Source: CAD feature listing. Evaluate the final solid. Frame: model axes, mm. Face numbers are marked on the shaded views. Give positions to 0.01 mm unless a question says otherwise; leave off trailing zeros. Write item = value, one per line.
from build123d import *

# Parameters (mm, degrees)
F1_DEPTH = 10
F2_DEPTH = 2.5
F3_R     = 5
F5_DEPTH = 12.501
F6_SIZE  = 1.5


# Not quite as in the source:
# - ends of sketch curves that miss each other by under 0.0002 mm in the source are joined


with BuildPart() as f1:
    # F0 (on Top) → F1 (new body, symmetric)
    with BuildSketch(Plane.XY):
        with BuildLine():
            ThreePointArc((-61.1270550584, 5.6233035221), (-64.3120758187, 10.4909176924), (-69.1094465162, 13.7807899309))
            ThreePointArc((-69.1094465162, 13.7807899309), (-89.3390658482, 4.5099582499), (-78.083775001, -14.6865061725))
            ThreePointArc((-78.083775001, -14.6865061725), (-72.0748340452, -14.7053930071), (-66.5406341793, -12.3643761411))
            ThreePointArc((-66.5406341793, -12.3643761411), (-71.7812655501, -10.9856736162), (-77.0668876123, -9.7910032715))
            ThreePointArc((-77.0668876123, -9.7910032715), (-84.570415019, 3.0066388333), (-71.0840021309, 9.1871932872))
            ThreePointArc((-71.0840021309, 9.1871932872), (-66.1610088951, 7.2502451775), (-61.1270550584, 5.6233035221))
        make_face()
        with BuildLine():
            ThreePointArc((-60.0331133604, 0), (-60.3091384465, 2.8643607899), (-61.1270550584, 5.6233035221))
            ThreePointArc((-61.1270550584, 5.6233035221), (-66.1610088951, 7.2502451775), (-71.0840021309, 9.1871932872))
            ThreePointArc((-71.0840021309, 9.1871932872), (-66.6817328669, 5.5004039718), (-65.0331133604, 0))
            ThreePointArc((-65.0331133604, 0), (-68.7219226752, -7.7568596826), (-77.0668877875, -9.791004115))
            ThreePointArc((-77.0668877875, -9.791004115), (-71.7812655501, -10.9856736162), (-66.5406341793, -12.3643761411))
            ThreePointArc((-66.5406341793, -12.3643761411), (-61.7593198612, -6.9861581818), (-60.0331133604, 0))
        make_face()
        with BuildLine():
            ThreePointArc((-13.906058302, 5.6233035221), (-8.2506059576, -12.5270707403), (10.6578947368, -10.5550594398))
            ThreePointArc((10.6578947368, -10.5550594398), (10.1646331199, -5.2877713941), (10, 0))
            ThreePointArc((10, 0), (-5.5004039718, -8.3513804935), (-3.9491112295, 9.1871932872))
            ThreePointArc((-3.9491112295, 9.1871932872), (-8.8721044653, 7.2502451775), (-13.906058302, 5.6233035221))
        make_face()
        with BuildLine():
            ThreePointArc((10.6578947368, -10.5550594398), (13.8720658348, -5.7066443269), (15, 0))
            ThreePointArc((15, 0), (8.2506059576, 12.5270707403), (-5.9236668442, 13.7807899309))
            ThreePointArc((-5.9236668442, 13.7807899309), (-10.7210375417, 10.4909176924), (-13.906058302, 5.6233035221))
            ThreePointArc((-13.906058302, 5.6233035221), (-8.8721044653, 7.2502451775), (-3.9491112295, 9.1871932872))
            ThreePointArc((-3.9491112295, 9.1871932872), (5.5004039718, 8.3513804935), (10, 0))
            ThreePointArc((10, 0), (10.1646331199, -5.2877713941), (10.6578947368, -10.5550594398))
        make_face()
        with BuildLine():
            ThreePointArc((26.5285242746, -50.3652361455), (23.527969189, -46.0081385383), (20.8042767721, -41.4728182632))
            ThreePointArc((20.8042767721, -41.4728182632), (9.3957138654, -44.3489563966), (3.5718338704, -54.5719647583))
            ThreePointArc((3.5718338704, -54.5719647583), (7.2428277606, -58.5580457504), (10.7722421784, -62.6700126379))
            ThreePointArc((10.7722421784, -62.6700126379), (12.3181130698, -48.4091450465), (26.5285242746, -50.3652361455))
        make_face()
        with BuildLine():
            ThreePointArc((33.4730565422, -56.2905580449), (32.7252146942, -51.6133806899), (30.5562581408, -47.4025751957))
            ThreePointArc((30.5562581408, -47.4025751957), (26.2662839534, -43.4739435732), (20.8042767721, -41.4728182632))
            ThreePointArc((20.8042767721, -41.4728182632), (23.527969189, -46.0081385383), (26.5285242746, -50.3652361455))
            ThreePointArc((26.5285242746, -50.3652361455), (27.9744953102, -53.1724398082), (28.4730565422, -56.2905580449))
            ThreePointArc((28.4730565422, -56.2905580449), (21.8636206345, -65.6982184946), (10.772241515, -62.6700131875))
            ThreePointArc((10.772241515, -62.6700131875), (7.2428277606, -58.5580457504), (3.5718338704, -54.5719647583))
            ThreePointArc((3.5718338704, -54.5719647583), (4.0929857429, -60.5582932532), (6.9218340013, -65.8597407588))
            ThreePointArc((6.9218340013, -65.8597407588), (23.5589026806, -70.4020487194), (33.4730565422, -56.2905580449))
        make_face()
        with BuildLine():
            ThreePointArc((-66.5406341793, -12.3643761411), (-72.0748340452, -14.7053930071), (-78.083775001, -14.6865061725))
            ThreePointArc((-78.083775001, -14.6865061725), (-31.2272831079, -33.0410645358), (6.9218340013, -65.8597407588))
            ThreePointArc((6.9218340013, -65.8597407588), (4.0929857429, -60.5582932532), (3.5718338704, -54.5719647583))
            ThreePointArc((3.5718338704, -54.5719647583), (-28.6485123869, -28.7573803523), (-66.5406341793, -12.3643761411))
        make_face()
        with BuildLine():
            ThreePointArc((-13.906058302, 5.6233035221), (-10.7210375417, 10.4909176924), (-5.9236668442, 13.7807899309))
            ThreePointArc((-5.9236668442, 13.7807899309), (-37.5165566802, 7.2783362288), (-69.1094465162, 13.7807899309))
            ThreePointArc((-69.1094465162, 13.7807899309), (-64.3120758187, 10.4909176924), (-61.1270550584, 5.6233035221))
            ThreePointArc((-61.1270550584, 5.6233035221), (-37.5165566802, 2.2783362288), (-13.906058302, 5.6233035221))
        make_face()
        with BuildLine():
            ThreePointArc((30.5562581408, -47.4025751957), (18.988489856, -24.9449458936), (15, 0))
            ThreePointArc((15, 0), (13.8720658348, -5.7066443269), (10.6578947368, -10.5550594398))
            ThreePointArc((10.6578947368, -10.5550594398), (14.237770472, -26.5040050119), (20.8042767721, -41.4728182632))
            ThreePointArc((20.8042767721, -41.4728182632), (26.2662839534, -43.4739435732), (30.5562581408, -47.4025751957))
        make_face()
    extrude(amount=F1_DEPTH, both=True)

    # F0 (on Top) → F2 (join, symmetric)
    with BuildSketch(Plane.XY):
        with BuildLine():
            ThreePointArc((20.8042767721, -41.4728182632), (14.237770472, -26.5040050119), (10.6578947368, -10.5550594398))
            ThreePointArc((10.6578947368, -10.5550594398), (-8.2506059576, -12.5270707403), (-13.906058302, 5.6233035221))
            ThreePointArc((-13.906058302, 5.6233035221), (-37.5165566802, 2.2783362288), (-61.1270550584, 5.6233035221))
            ThreePointArc((-61.1270550584, 5.6233035221), (-60.3091384465, 2.8643607899), (-60.0331133604, 0))
            ThreePointArc((-60.0331133604, 0), (-61.7593198612, -6.9861581818), (-66.5406341793, -12.3643761411))
            ThreePointArc((-66.5406341793, -12.3643761411), (-28.6485123869, -28.7573803523), (3.5718338704, -54.5719647583))
            ThreePointArc((3.5718338704, -54.5719647583), (9.3957138654, -44.3489563966), (20.8042767721, -41.4728182632))
        make_face()
    extrude(amount=F2_DEPTH, both=True)

    # F3
    f3_edges = [f1.edges().sort_by_distance(p)[0] for p in [
        (14.23777, -26.504005, 2.5),
        (-8.250606, -12.527071, 2.5),
        (-37.516557, 2.278336, 2.5),
        (-60.669521, -4.322872, 2.5),
        (-28.648512, -28.75738, 2.5),
        (9.395714, -44.348956, 2.5),
        (14.23777, -26.504005, -2.5),
        (-8.250606, -12.527071, -2.5),
        (-37.516557, 2.278336, -2.5),
        (-60.669521, -4.322872, -2.5),
        (-28.648512, -28.75738, -2.5),
        (9.395714, -44.348956, -2.5),
    ]]
    fillet(f3_edges, radius=F3_R)

    # F4 (on face) → F5 (cut, through all)
    with BuildSketch(Plane.XY.offset(2.5)):
        with BuildLine():
            ThreePointArc((4.7631578947, -22.5013849989), (-12.650929135, -19.2081751351), (-22.5534813546, -4.5100419942))
            ThreePointArc((-22.5534813546, -4.5100419942), (-37.5165566802, -5.7216637712), (-52.4796320058, -4.5100419942))
            ThreePointArc((-52.4796320058, -4.5100419942), (-52.9254779245, -6.3444822825), (-53.5202661907, -8.1361788731))
            ThreePointArc((-53.5202661907, -8.1361788731), (-24.5224799443, -21.9034868397), (1.2149484666, -41.0866866415))
            ThreePointArc((1.2149484666, -41.0866866415), (4.7912073526, -37.8025348204), (8.9772080845, -35.3423155872))
            ThreePointArc((8.9772080845, -35.3423155872), (6.6366194576, -28.9984996013), (4.7631578947, -22.5013849989))
        make_face()
    extrude(amount=-F5_DEPTH, mode=Mode.SUBTRACT)

    # F6
    f6_edges = [f1.edges().sort_by_distance(p)[0] for p in [
        (-84.570415, 3.006639, 10),
        (3.949111, -9.187193, 10),
        (12.318113, -48.409145, 10),
    ]]
    chamfer(f6_edges, length=F6_SIZE)


solid = f1.part
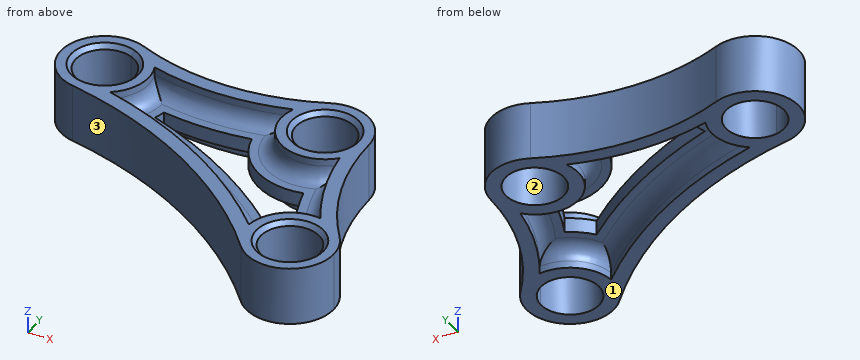
1) Cut plane A-A (z = -4.5). State how many separate pieces and enclosed holes the cut face has, then the cut area to 3 significant figures.
Computed:
separate_pieces = 1
enclosed_holes = 4
area = 2,310 mm²
2) Draft query along X for the marked faces 1, 2 and 3. Return one class per face: pulls with the +X half, pulls with the -X half, needs draft (parallel to the pull), parting line crosses it, or undercut.
Computed:
face_1 = needs draft
face_2 = undercut
face_3 = pulls with the -X half
3) Contact query for flat-ended pins moving along their axis: pin 1 (5 mm diameter, centred on x = -20.5, y = -21.5, fed in from +Z); pin 2 (12 mm diameter, centred on x = -75.03, y = 0, fed in from -Z); pin 3 (12 mm diameter, centred on x = -26.5, z = 4.5, fed in from +Y); pin 4 (4 mm diameter, centred on x = -61, z = 6, fed in from +Y). Output: stop coordinate, or through.
Computed:
pin_1 = 2.5
pin_2 = through
pin_3 = 9.11
pin_4 = 11.45
4) Material intervals for L1, parallel to Y at x = 0, z = -1.25; L2, parallel to Y at x = 0, z = -3.75; L3, parallel to Z at x = -19, y = -11.5, sorted ascending.
Computed:
L1 = -58.07 to -39.99, -23 to -10, 10 to 15
L2 = -58.07 to -48.59, -16.69 to -10, 10 to 15
L3 = -2.5 to 2.5
